The figure shows three views and two pictorial views of one solid part (mm, origin at its lowest corner). Answer the questions. Give positions to 0.01 mm unless a question says otherwise; leave off trailing zeros. Order: outer loops, then holes, each group sorted by start corner. A loop starts at its lowest first (then second) coordinate and runs counter-clockwise, first axis right, second up. Notation, with made-up numbers: (-19, 30) - (38, 30) arc R20 cw to (38, 45) - close; hole circle Ø10 at (-6, -3). An arc over 180 degrees is marked (long way). Answer as a JSON object with one key per item and string values. Group by question number.
Q1. A cutting plane is placed at A-A, the plane x = 1.55. Give the vertices of the cut face in (y, z).
Q2. A cutting plane is placed at C-C, the plane z = 126.5. Give the vertices of the cut face in (x, y).
Q3. Consider line 1 (Z direction, x = 4.85, y = 26); line 2 (Y direction, x = 3.1, z = 24.5). Determine where each line is inside the solid, lowest interval first.
Q4. Given pin 1 (2.5 mm diameter, centred on x = 3, y = 1.5, fed in from +Z); pin 2 (1.5 mm diameter, centred on x = 2, z = 141.5, fed in from -Y); pin 3 (1.5 mm diameter, centred on x = 3.5, y = 31, fed in from -Z), each flat-ended and moving along its own axis, determine where each tip first touches the part or whether it passes through.
Q5. A cutting plane is placed at B-B, the plane y = 56. Give the vertices of the cut face in (x, z), and give its area (3 significant figures).
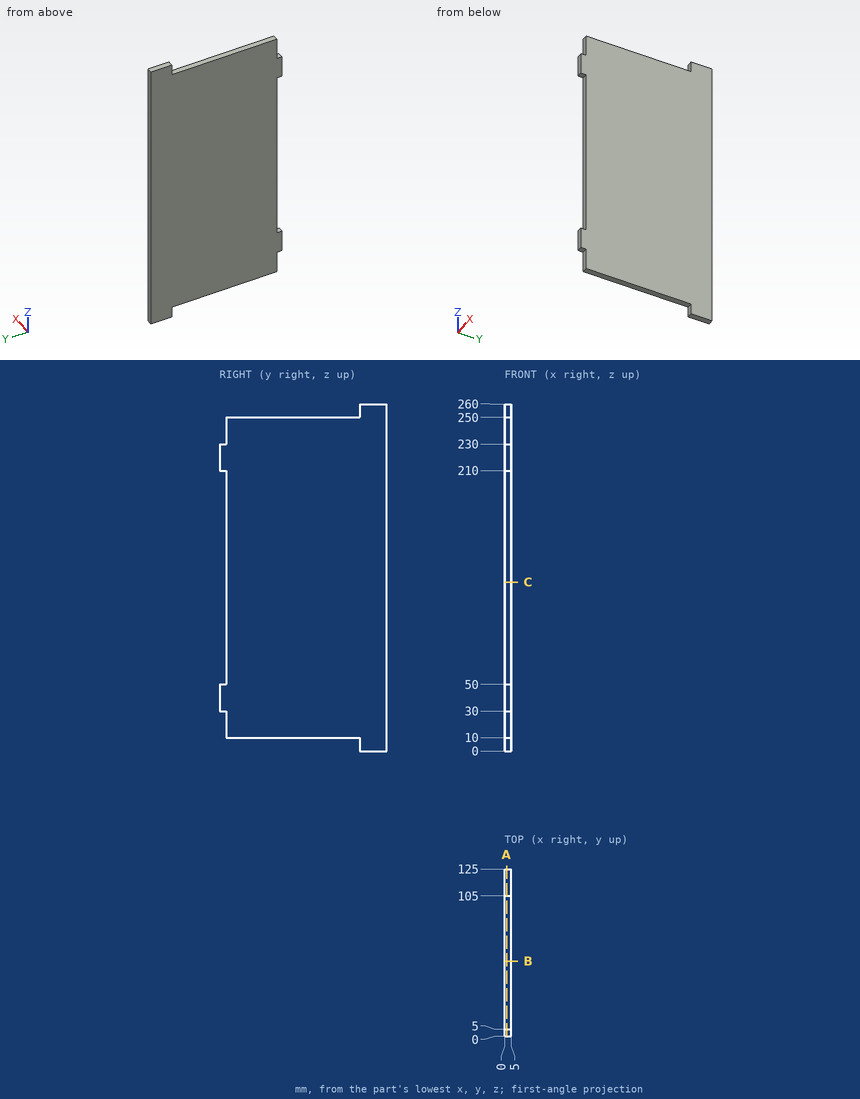
Reply:
{
 "1": {"outline": "(0, 30) - (5, 30) - (5, 10) - (105, 10) - (105, 0) - (125, 0) - (125, 260) - (105, 260) - (105, 250) - (5, 250) - (5, 230) - (0, 230) - (0, 210) - (5, 210) - (5, 50) - (0, 50) - close"},
 "2": {"outline": "(0, 5) - (5, 5) - (5, 125) - (0, 125) - close"},
 "3": {"line 1": "z = 10 to 250", "line 2": "y = 5 to 125"},
 "4": {"pin 1": "stops at z = 230", "pin 2": "stops at y = 5", "pin 3": "stops at z = 10"},
 "5": {"outline": "(0, 10) - (5, 10) - (5, 250) - (0, 250) - close", "area": "1,200 mm^2"}
}
